Build history of the part. All positions in model axes, mm. A direction names the side the tool comes from. Round coordinates to 2 decimals unless told otherwise and drop trailing zeros. Loops run counter-clockwise (first coordinate to the right, second up) from the corner with the lowest first, then second, coordinate; pieces in that order, holes last. Notation, with made-up numbers: (34, 29.25) - (83, 29.25) arc R9 cw to (83, 41.25) - close; hole circle Ø10 at (16.25, 85.5). An arc over 180 degrees is marked (long way). Use one line per item in the form item = value. Start each with the question number.
Q1. Drill centre lines: line 1 (Y direction, x = 53.5, z = 13.5) (3 decimals); line 2 (X direction, y = 205.5, z = 104.5) (3 decimals). Where is each one in solid material? Low to high.
Q2. 3-axis set-ups, long thin cutter, end or side, ignore diameter. For faces 1 (the face through (247.65, 125, 114)), 2 (the face through (125, 9.525, 67)), 3 (the face through (245.84, 245.74, 114.48)), 4 (the face through (8.16, 8.26, 114.48)): which of +Z, -Z, +X, -X, +Y, -Y reach the whole face in a straight line?
Q3. Saw through at B-B (z = 23.5). Give the cut face in (x, y) (3 decimals).
Q4. Saw through at D-D (z = 106). Give the cut face in (x, y) (3 decimals), then the cut area to 3 significant figures.
Q5. Pin check, flat tips, straight feed: pin 1 (7.5 mm diameter, centred on x = 145, z = 113.5, fed in from -Y); pin 2 (8 mm diameter, centred on x = 200, y = 44, fed in from +Z) (3 decimals); pin 3 (1.5 mm diameter, centred on y = 117, z = 107, fed in from +X); pin 4 (4 mm diameter, centred on x = 98.5, y = 158.5, fed in from -Z). Stop position of each tip, or through.
Q6. Saw through at A-A (x = 191). Give the cut face in (y, z) (3 decimals).
Q7. Mould opens along X. For faces 5 (the face through (129, 247.65, 114)), 6 (the face through (8.26, 245.84, 114.48)), 7 (the face through (244.475, 125, 67)) say: released by +X, released by -X, zero draft, split by the parting line, or undercut.
```python
from build123d import *

# Parameters (mm, degrees)
SKETCH2_W          = 254
SKETCH2_H          = 254
EXTRUDE1_DEPTH     = 127
FILLET1_R          = 12.7
SHELL1_T           = -9.525
CUT_EXTRUDE1_DEPTH = 25.4


with BuildPart() as part:
    # Sketch2 → Extrude1 (new body)
    with BuildSketch(Plane.XY):
        with Locations((127, 127)):
            Rectangle(SKETCH2_W, SKETCH2_H)
    extrude(amount=EXTRUDE1_DEPTH)

    # Fillet1
    fillet1_edges = [part.edges().sort_by_distance(p)[0] for p in [
        (0, 254, 63.5),
        (254, 254, 63.5),
        (254, 0, 63.5),
        (0, 0, 63.5),
    ]]
    fillet(fillet1_edges, radius=FILLET1_R)

    # Shell1
    shell1_openings = [part.faces().sort_by_distance(p)[0] for p in [
        (127, 127, 127),
    ]]
    offset(amount=SHELL1_T, openings=shell1_openings, kind=Kind.INTERSECTION)

    # Sketch3 → Cut-Extrude1 (cut)
    with BuildSketch(Plane.XY.offset(127)):
        with BuildLine():
            Line((0, 241.3), (0, 12.7))
            ThreePointArc((0, 12.7), (3.719743879, 3.719743879), (12.7, 0))
            Line((12.7, 0), (241.3, 0))
            ThreePointArc((241.3, 0), (250.280256121, 3.719743879), (254, 12.7))
            Line((254, 12.7), (254, 241.3))
            ThreePointArc((254, 241.3), (250.280256121, 250.280256121), (241.3, 254))
            Line((241.3, 254), (12.7, 254))
            ThreePointArc((12.7, 254), (3.719743879, 250.280256121), (0, 241.3))
        make_face()
        with BuildLine():
            Line((6.35, 241.3), (6.35, 12.7))
            ThreePointArc((6.35, 12.7), (8.209871939, 8.209871939), (12.7, 6.35))
            Line((12.7, 6.35), (241.3, 6.35))
            ThreePointArc((241.3, 6.35), (245.790128061, 8.209871939), (247.65, 12.7))
            Line((247.65, 12.7), (247.65, 241.3))
            ThreePointArc((247.65, 241.3), (245.790128061, 245.790128061), (241.3, 247.65))
            Line((241.3, 247.65), (12.7, 247.65))
            ThreePointArc((12.7, 247.65), (8.209871939, 245.790128061), (6.35, 241.3))
        make_face(mode=Mode.SUBTRACT)
    extrude(amount=-CUT_EXTRUDE1_DEPTH, mode=Mode.SUBTRACT)


solid = part.part
```
Report:
q1.line_1 = 0 to 9.525, 244.475 to 254
q1.line_2 = 6.35 to 9.525, 244.475 to 247.65
q2.face_1 = +Z, +X, +Y, -Y
q2.face_2 = +Z
q2.face_3 = +Z, +X, +Y
q2.face_4 = +Z, -X, -Y
q3.outline = (0, 12.7) arc R12.7 ccw to (12.7, 0) - (241.3, 0) arc R12.7 ccw to (254, 12.7) - (254, 241.3) arc R12.7 ccw to (241.3, 254) - (12.7, 254) arc R12.7 ccw to (0, 241.3) - close; hole (9.525, 12.7) arc R3.175 ccw to (12.7, 9.525) - (241.3, 9.525) arc R3.175 ccw to (244.475, 12.7) - (244.475, 241.3) arc R3.175 ccw to (241.3, 244.475) - (12.7, 244.475) arc R3.175 ccw to (9.525, 241.3) - close
q4.outline = (6.35, 12.7) arc R6.35 ccw to (12.7, 6.35) - (241.3, 6.35) arc R6.35 ccw to (247.65, 12.7) - (247.65, 241.3) arc R6.35 ccw to (241.3, 247.65) - (12.7, 247.65) arc R6.35 ccw to (6.35, 241.3) - close; hole (9.525, 12.7) arc R3.175 ccw to (12.7, 9.525) - (241.3, 9.525) arc R3.175 ccw to (244.475, 12.7) - (244.475, 241.3) arc R3.175 ccw to (241.3, 244.475) - (12.7, 244.475) arc R3.175 ccw to (9.525, 241.3) - close
q4.area = 3,000 mm²
q5.pin_1 = 6.35
q5.pin_2 = 9.525
q5.pin_3 = 247.65
q5.pin_4 = 0
q6.outline = (0, 0) - (254, 0) - (254, 101.6) - (247.65, 101.6) - (247.65, 127) - (244.475, 127) - (244.475, 9.525) - (9.525, 9.525) - (9.525, 127) - (6.35, 127) - (6.35, 101.6) - (0, 101.6) - close
q7.face_5 = zero draft
q7.face_6 = released by -X
q7.face_7 = undercut
